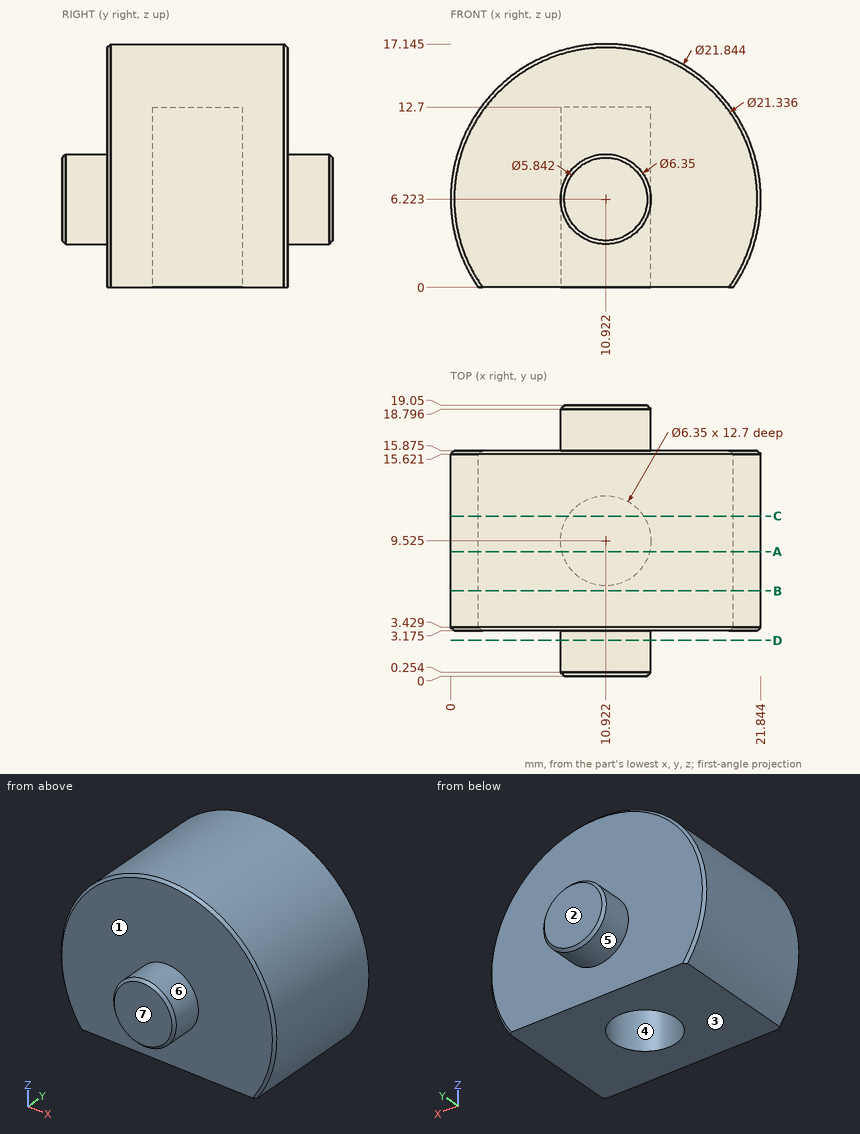
Geometry check sheet. Reference: drawing and pictorial views, mm from the part's lowest x, y, z. A direction names the side the tool comes from. Give positions to 0.01 mm unless a question says otherwise; leave off trailing zeros. Order: outer loops, then holes, each group sorted by start corner. A loop starts at its lowest first (then second) coordinate and runs counter-clockwise, first axis right, second up.
1. Section check A-A, the plane y = 8.75. Enter the section's corners in (x, z), and give its area (3 significant figures).
2. Gauge pin test, flat ends, axial feed: pin 1 Ø1 at (y, z) = (14, 11.5) entering from +X; pin 2 Ø8 at (x, z) = (5.5, 14) entering from -Y (3 decimals); pin 3 Ø2 at (x, z) = (17.5, 9) entering from +Y (3 decimals). Record the tip position at first contact, or that the pin passes through.
3. Release check for a two-part mould opening along Y. For the marked faces 1, 2, 3 and 4 record: pulls with the +Y half, pulls with the -Y half, needs draft (parallel to the pull), parting line crosses it, or undercut.
4. Section check D-D, the plane y = 2.5. Enter the section's corners in (x, z) (3 decimals), and give its area (3 significant figures).
5. Thickness scan on L1, parallel to Y at x = 15.5, z = 11.75 (3 decimals); L2, parallel to Y at x = 12.5, z = 11 (3 decimals); L3, parallel to Y at x = 8.25, z = 5. Record the ranges inside material, lowest first.
6. Section check B-B, the plane y = 6. Enter the section's corners in (x, z).
7. Access from +Z, -Z, +X, -X, +Y, -Y to the whole of each face (thin tool, end or side, straight path). Record for the marked faces 5, 6 and 7.
8. Section check C-C, the plane y = 11.25. Enter the section's corners in (x, z).
Values follow:
1. outline: (1.95, 0) - (7.84, 0) - (7.84, 12.7) - (14, 12.7) - (14, 0) - (19.9, 0) arc R10.92 ccw (long way) to start
1. area: 237 mm2
2. pin 1: stops at x = 20.74
2. pin 2: stops at y = 3.175
2. pin 3: stops at y = 15.875
3. face 1: pulls with the -Y half
3. face 2: pulls with the +Y half
3. face 3: needs draft
3. face 4: undercut
4. outline: circle Ø6.35 at (10.922, 6.223)
4. area: 31.7 mm2
5. L1: y = 3.175 to 15.875
5. L2: y = 3.175 to 6.77, 12.28 to 15.875
5. L3: y = 0.02 to 7.81, 11.24 to 19.03
6. outline: (1.95, 0) - (19.9, 0) arc R10.92 ccw (long way) to start
7. face 5: +Y
7. face 6: -Y
7. face 7: +Z, -Z, +X, -X, -Y
8. outline: (1.95, 0) - (8.26, 0) - (8.26, 12.7) - (13.59, 12.7) - (13.59, 0) - (19.9, 0) arc R10.92 ccw (long way) to start
